from build123d import *

# Parameters (mm, degrees)
F2_R     = 4.7625
F3_DEPTH = 9.525
F4_R     = 1.5875
F5_DEPTH = 25.4


with BuildPart() as f1:
    # F0 (on Front) → F1 (revolve)
    with BuildSketch(Plane.XZ):
        with BuildLine():
            Line((0, 54.107483), (0, 0))
            Line((0, 0), (19.858597, 16.692733))
            Line((19.858597, 16.692733), (19.858597, 30.219605))
            Line((19.858597, 30.219605), (31.658631, 30.219605))
            Line((31.658631, 30.219605), (31.658631, 42.307448))
            ThreePointArc((31.658631, 42.307448), (20.795094, 33.8991), (7.48295, 30.50741))
            Line((7.48295, 30.50741), (7.48295, 54.107483))
            Line((7.48295, 54.107483), (0, 54.107483))
        make_face()
    revolve(axis=Axis((0, 0, 27.053742), (0, 0, 1)))

    # F2 (on face) → F3 (cut)
    with BuildSketch(Plane.XY.offset(54.107483)):
        Circle(F2_R)
    extrude(amount=-F3_DEPTH, mode=Mode.SUBTRACT)

    # F4 (on Top) → F5 (cut)
    with BuildSketch(Plane.XY):
        Circle(F4_R)
    extrude(amount=F5_DEPTH, mode=Mode.SUBTRACT)


solid = f1.part
Part model, mm, in its own coordinate system. A direction names the side the tool comes from. Give positions to 0.01 mm unless a question says otherwise; leave off trailing zeros. Write each loop counter-clockwise with the first axis right and the second up, starting at its lowest first coordinate (ties: lowest second). Pieces come first, ordered by that corner, then holes.
1) Cut at D-D on z = 9. Write the cut outline in (x, y) (1 decimal).
Resolved:
outline: circle Ø21.4 at (0, 0); hole circle Ø3.2 at (0, 0)
2) Probe L1, parallel to Y at x = 0, z = 49; L2, parallel to Y at x = -21, z = 37.5; L3, parallel to X at y = 3, z = 39.5. List the from-to ranges inside material, lowest first.
Resolved:
L1: y = -7.48 to -4.76, 4.76 to 7.48
L2: y = -23.69 to -16.33, 16.33 to 23.69
L3: x = -31.52 to -28.81, -6.86 to 6.86, 28.81 to 31.52
3) Cut at A-A on z = 23.5. Write the cut outline in (x, y) (1 decimal).
Resolved:
outline: circle Ø39.7 at (0, 0); hole circle Ø3.2 at (0, 0)
4) Which spindle directions (+Z, -Z, +X, -X, +Y, -Y) get a long thin tool onto all of the face, cutting with end or side? Do faces 1 (the face through (-25.123, -19.264, 36.348)), 2 (the face through (-3.78, -2.9, 49.41)). Say none if no direction does.
Resolved:
face 1: +Z, -Z
face 2: +Z
5) Cut at C-C on z = 34.5. State how many separate pieces and enclosed holes the cut face has, then the cut area to 3 significant figures.
Resolved:
separate pieces: 2
enclosed holes: 1
area: 1,810 mm2
6) Two-plate mould, pull along X, no slides. Class faces 3 (the face through (-4.305, -19.386, 23.551)), 4 (the face through (0, 0, 25.4)), 5 (the face through (-0.34, -1.55, 13.2)), 6 (the face through (15, -14, 30.22)): released by +X, released by -X, zero draft, split by the parting line, or undercut.
Resolved:
face 3: split by the parting line
face 4: undercut
face 5: undercut
face 6: zero draft
7) Cut at B-B on z = 29. Write the cut outline in (x, y).
Resolved:
outline: circle Ø39.72 at (0, 0)
8) Pin check, flat tips, straight feed: pin 1 (2 mm diameter, centred on y = 20, z = 34, fed in from -X); pin 2 (6 mm diameter, centred on x = -19.5, y = 18, fed in from -Z); pin 3 (2 mm diameter, centred on y = 10, z = 12, fed in from -X). Stop position of each tip, or through.
Resolved:
pin 1: stops at x = -25.32
pin 2: stops at z = 30.22
pin 3: stops at x = -12
